Source: CAD feature listing. Evaluate the final solid. Frame: model axes, mm. Face numbers are marked on the shaded views. A direction names the side the tool comes from. Give positions to 0.01 mm unless a question says otherwise; leave off trailing zeros. Loops run counter-clockwise (first coordinate to the right, second up) from the corner with the lowest first, then second, coordinate; pieces in that order, holes last. Notation, with made-up numbers: (-16, -2) - (20, -2) arc R25 ccw to (20, 37) - close; hole circle Ø8 at (-28.75, 45). An arc over 180 degrees is marked (long way). Write each question's results on one line, items separated by ' | '. Start each with the question number.
(1) Pull-direction query (X, two-part tool) for the marked faces 3, 4 and 5; classes: pulls with the +X half, pulls with the -X half, needs draft (parallel to the pull), parting line crosses it, or undercut.
(2) Reachability of the marked faces 1 and 2 from +Z, -Z, +X, -X, +Y, -Y: full face, straight path, thin tool, end or side. Return the list, or none.
(3) Material intervals for line 1 along X through (y, z) = (-1.55, -5.25); line 2 along Y through (x, z) = (0.5, -1.5); line 3 along Z through (x, y) = (8.25, -2.65), sorted ascending. Write a range as [from, to].
(4) Cut plane B-B on z = -4. Return the cut outline in (x, y), then the cut area to 3 significant figures.
(5) Cut plane A-A on x = -8. Return the cut outline in (y, z).
(6) Cut plane D-D on z = 9.5. Return the cut outline in (x, y), then the cut area to 3 significant figures.
(7) Contact query for flat-ended pins moving along their axis: pin 1 (0.6 mm diameter, centred on y = -2.5, z = 2, fed in from +X); pin 2 (1 mm diameter, centred on x = -4.5, y = -2, fed in from -Z); pin 3 (0.6 mm diameter, centred on x = 1, y = -2, fed in from +Z). Output: stop coordinate, or through.
(8) Cut plane C-C on y = -1.3. Return the cut outline in (x, z).
from build123d import *

# Parameters (mm, degrees)
SKETCH1_W           = 22
SKETCH1_H           = 22
BOSS_EXTRUDE1_DEPTH = 1
BOSS_EXTRUDE2_DEPTH = 2


with BuildPart() as part:
    # Sketch1 → Boss-Extrude1 (new, symmetric)
    with BuildSketch(Plane(origin=(0, 0, 0), x_dir=(1, 0, 0), z_dir=(0, 1, 0))):
        Rectangle(SKETCH1_W, SKETCH1_H)
    extrude(amount=BOSS_EXTRUDE1_DEPTH, both=True)

    # Sketch2 → Boss-Extrude2 (add)
    with BuildSketch(Plane.XZ.offset(1)):
        Polygon((-7.25, 7.25), (-7.25, 8.75), (-8.75, 8.75), (-8.75, -8.75), (8.75, -8.75), (8.75, 8.75), (7.25, 8.75), (7.25, 7.25), (7.25, -7.25), (-7.25, -7.25), align=None)
    extrude(amount=BOSS_EXTRUDE2_DEPTH)


solid = part.part
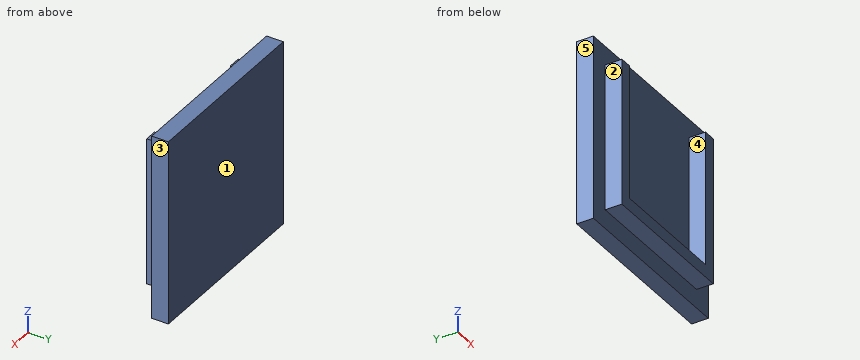
Ans:
1) face 3: pulls with the +X half | face 4: undercut | face 5: pulls with the -X half
2) face 1: +Z, -Z, +X, -X, +Y | face 2: +Z, -Z, -X, -Y
3) line 1: [-8.75, -7.25], [7.25, 8.75] | line 2: [-1, 1] | line 3: [-8.75, 8.75]
4) outline: (-11, -1) - (-8.75, -1) - (-8.75, -3) - (-7.25, -3) - (-7.25, -1) - (7.25, -1) - (7.25, -3) - (8.75, -3) - (8.75, -1) - (11, -1) - (11, 1) - (-11, 1) - close | area: 50.0 mm^2
5) outline: (-3, -8.75) - (-1, -8.75) - (-1, -11) - (1, -11) - (1, 11) - (-1, 11) - (-1, 8.75) - (-3, 8.75) - close
6) outline: (-11, -1) - (11, -1) - (11, 1) - (-11, 1) - close | area: 44.0 mm^2
7) pin 1: x = 8.75 | pin 2: z = -8.75 | pin 3: z = -7.25
8) outline: (-8.75, -8.75) - (8.75, -8.75) - (8.75, 8.75) - (7.25, 8.75) - (7.25, -7.25) - (-7.25, -7.25) - (-7.25, 8.75) - (-8.75, 8.75) - close
